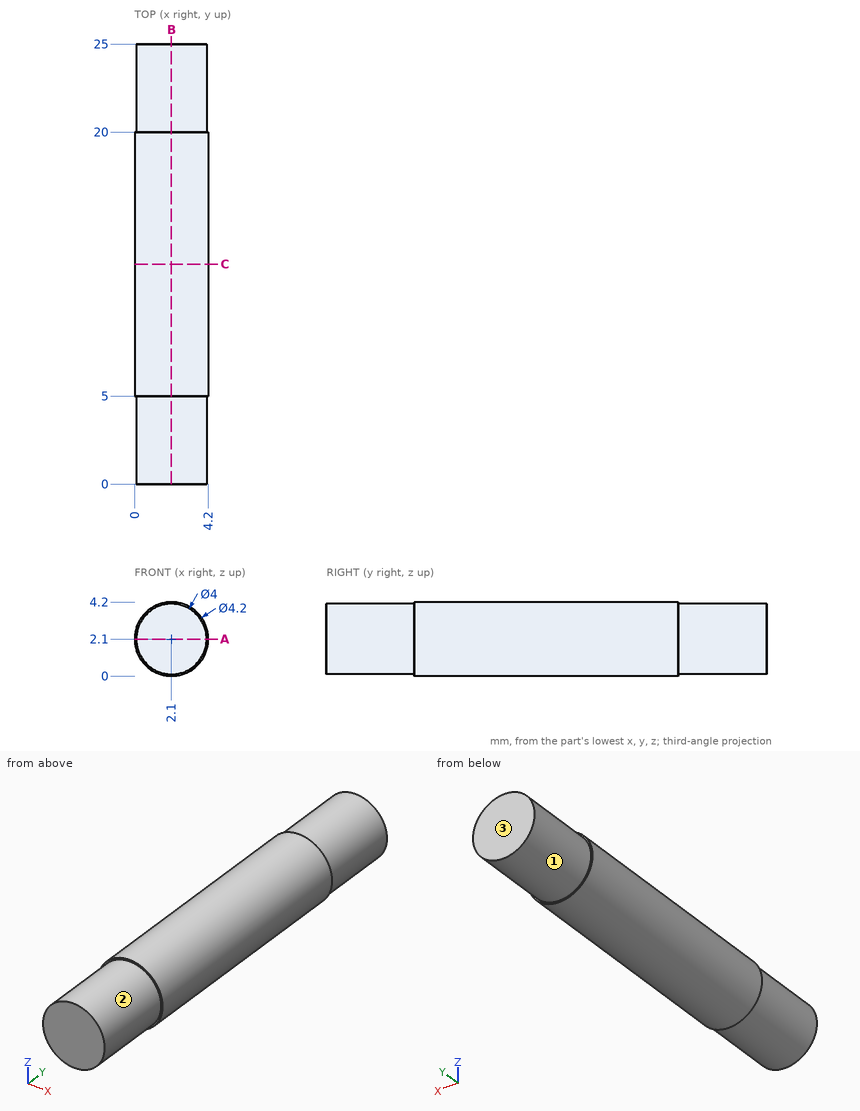
Could you check a few things on this drawing? It's one solid part, dimensions in mm from its lowest x, y, z. A direction names the side the tool comes from. Coordinates: 2 decimals unless noted, no trailing zeros. Order: outer loops, then holes, each group sorted by start corner. A loop starts at its lowest first (then second) coordinate and runs counter-clockwise, first axis right, second up.
1. If we section it at C-C (y = 12.5): Please give me the cut outline in (x, z), then the cut area to 3 significant figures.
2. I'm going to push flat-ended pins straight in: pin 1 (2 mm diameter, centred on y = 19, z = 1.5, fed in from -X); pin 2 (1.5 mm diameter, centred on y = 9.5, z = 1, fed in from +X). Where does each tip first touch, or does it pass through?
3. For the marked faces 1, 2 and 3, which set-ups out of +Z, -Z, +X, -X, +Y, -Y let a thin tool reach every point of the face, with its end or its side?
4. If we section it at A-A (z = 2.1): Please give me the cut outline in (x, y).
5. If we section it at B-B (x = 2.1): Please give me the cut outline in (y, z).
6. I need wall thicknesses on line 1 (Y direction, x = 1.15, z = 0.3); line 2 (Z direction, x = 3.5, y = 8.75); line 3 (X direction, y = 10.25, z = 0.6). Which ranges of each line are inside material? Lowest first, please.
Entries:
1. outline: circle Ø4.2 at (2.1, 2.1)
1. area: 13.9 mm2
2. pin 1: stops at x = 0
2. pin 2: stops at x = 4.17
3. face 1: +Y
3. face 2: -Y
3. face 3: +Z, -Z, +X, -X, +Y
4. outline: (0, 5) - (0.1, 5) - (0.1, 0) - (4.1, 0) - (4.1, 5) - (4.2, 5) - (4.2, 20) - (4.1, 20) - (4.1, 25) - (0.1, 25) - (0.1, 20) - (0, 20) - close
5. outline: (0, 0.1) - (5, 0.1) - (5, 0) - (20, 0) - (20, 0.1) - (25, 0.1) - (25, 4.1) - (20, 4.1) - (20, 4.2) - (5, 4.2) - (5, 4.1) - (0, 4.1) - close
6. line 1: y = 5 to 20
6. line 2: z = 0.53 to 3.67
6. line 3: x = 0.63 to 3.57
